Part model, mm, in its own coordinate system. Face numbers are marked on the shaded views. A direction names the side the tool comes from. Round coordinates to 2 decimals unless told otherwise and drop trailing zeros. Write each loop counter-clockwise with the first axis right and the second up, starting at its lowest first coordinate (ties: lowest second). Pieces come first, ordered by that corner, then holes. Notation, with made-up numbers: M -5.75,16 L 33.25,16 A30 ccw 33.25,38 Z; hole C 9.25,72.25 d7. An arc over 180 degrees is marked long. Use a Markdown table: item, result. Add a question column.
1) Slice it at D-D on y = 18. Write the cut outline in (x, z).
2) Drop flat-ended pins along their axis: P1, Ø1.5, axis at y = 25, z = 8, coming from the -X side; P2, Ø10, axis at y = -3.5, z = 8, coming from the +X side; P3, Ø12, axis at x = 19, y = 10, coming from the +Z side; P4, Ø1.5, axis at x = 31, z = 10.5, coming from the +Y side. Give the stop position or say it passes through.
3) Slice it at C-C on z = 26. Write the cut outline in (x, y), plus the area to 3 significant figures.
4) Two-plate mould, pull along Z, no slides. Class the marked faces 1, 2, 3 and 4: released by +Z, released by -Z, zero draft, split by the parting line, or undercut.
5) Slice it at A-A on z = 2.5. Write the cut outline in (x, y).
6) Slice it at B-B on y = 2. Write the cut outline in (x, z).
7) Which spindle directions (+Z, -Z, +X, -X, +Y, -Y) get a long thin tool onto all of the face, cutting with end or side? Do the marked faces 5, 6 and 7. Say none if no direction does.
8) Wall check: probe 1 along Z at (x, y) = (0, 0); probe 2 along Z at (x, y) = (0, 29.75); probe 3 along X at (y, z) = (-4.25, 8). Give the ranges that are in metal, low to high.
```python
from build123d import *

# Parameters (mm, degrees)
BOSS_EXTRUDE2_DEPTH       = 28
SKETCH5_R                 = 6
CUT_EXTRUDE1_DEPTH        = 24
CUT_EXTRUDE3_DEPTH        = 22
HOLE1_START               = 23.196151292
HOLE1_OUTLINE_R           = 3
HOLE1_DEPTH               = 12.803848708
HOLE1_START_2             = 32
HOLE1_2_OUTLINE_R         = 5
HOLE1_2_OUTLINE_R_2       = 3
HOLE1_2_DEPTH             = 4
F_6_0MM_DOWEL_HOLE2_D     = 6
F_6_0MM_DOWEL_HOLE2_DEPTH = 16
F_6_0MM_DOWEL_HOLE2_TIP   = 1.802581857
FILLET1_R                 = 3
SKETCH19_W                = 64
SKETCH19_H                = 4
BOSS_EXTRUDE3_DEPTH       = 2


# Read off the part's stored shape, not the designer's step: Hole1
with BuildPart() as part:
    # Sketch2 → Boss-Extrude2 (new body)
    with BuildSketch(Plane.XY):
        Polygon((0, -9), (-8, -9), (-8, 0), (-32, 0), (-32, 36), (32, 36), (32, 0), (8, 0), (8, -9), align=None)
    extrude(amount=BOSS_EXTRUDE2_DEPTH)

    # Sketch5 → Cut-Extrude1 (cut)
    with BuildSketch(Plane.XY):
        with Locations((0, 18)):
            Circle(SKETCH5_R)
    extrude(amount=CUT_EXTRUDE1_DEPTH, mode=Mode.SUBTRACT)

    # Sketch6 → Cut-Extrude3 (cut)
    with BuildSketch(Plane(origin=(0, 0, 0), x_dir=(-1, 0, 0), z_dir=(0, 0, -1))):
        with BuildLine():
            Line((-32, 36), (-32, 10))
            Line((-32, 10), (-27.5, 10))
            Line((-27.5, 10), (-14.77335007, 28.283390866))
            ThreePointArc((-14.77335007, 28.283390866), (-8.333635583, 33.954639387), (2.5e-08, 36))
            Line((2.5e-08, 36), (-32, 36))
        make_face()
        with BuildLine():
            Line((32, 36), (2.5e-08, 36))
            ThreePointArc((2.5e-08, 36), (8.333635604, 33.954639376), (14.77335007, 28.283390866))
            Line((14.77335007, 28.283390866), (27.5, 10))
            Line((27.5, 10), (32, 10))
            Line((32, 10), (32, 36))
        make_face()
    extrude(amount=-CUT_EXTRUDE3_DEPTH, mode=Mode.SUBTRACT)

    # Hole1 outline → Hole1 (cut)
    with BuildSketch(Plane(origin=(0, 0, 0), x_dir=(1, 0, 0), z_dir=(0, 1, 0)).offset(HOLE1_START)):
        with Locations((0, -11)):
            Circle(HOLE1_OUTLINE_R)
    extrude(amount=HOLE1_DEPTH, mode=Mode.SUBTRACT)

    # Hole1 2 outline → Hole1 2 (cut)
    with BuildSketch(Plane(origin=(0, 0, 0), x_dir=(1, 0, 0), z_dir=(0, 1, 0)).offset(HOLE1_START_2)):
        with Locations((0, -11)):
            Circle(HOLE1_2_OUTLINE_R)
        with Locations((0, -11)):
            Circle(HOLE1_2_OUTLINE_R_2, mode=Mode.SUBTRACT)
    extrude(amount=HOLE1_2_DEPTH, mode=Mode.SUBTRACT)

    # Ø6.0mm Dowel Hole2
    with Locations(Plane(origin=(0, -9, 0), x_dir=(-1, 0, 0), z_dir=(0, -1, 0))):
        with Locations((0, -20), (0, -8)):
            Hole(F_6_0MM_DOWEL_HOLE2_D / 2, depth=F_6_0MM_DOWEL_HOLE2_DEPTH)
            with Locations((0, 0, -(F_6_0MM_DOWEL_HOLE2_DEPTH + F_6_0MM_DOWEL_HOLE2_TIP / 2))):  # 118° drill point
                Cone(0, F_6_0MM_DOWEL_HOLE2_D / 2, F_6_0MM_DOWEL_HOLE2_TIP, mode=Mode.SUBTRACT)

    # Fillet1
    fillet1_edges = [part.edges().sort_by_distance(p)[0] for p in [
        (27.5, 10, 11),
        (-27.5, 10, 11),
    ]]
    fillet(fillet1_edges, radius=FILLET1_R)

    # Sketch19 → Boss-Extrude3 (add)
    with BuildSketch(Plane.XY.offset(28)):
        with Locations((0, 30)):
            Rectangle(SKETCH19_W, SKETCH19_H)
    extrude(amount=BOSS_EXTRUDE3_DEPTH)


solid = part.part
```
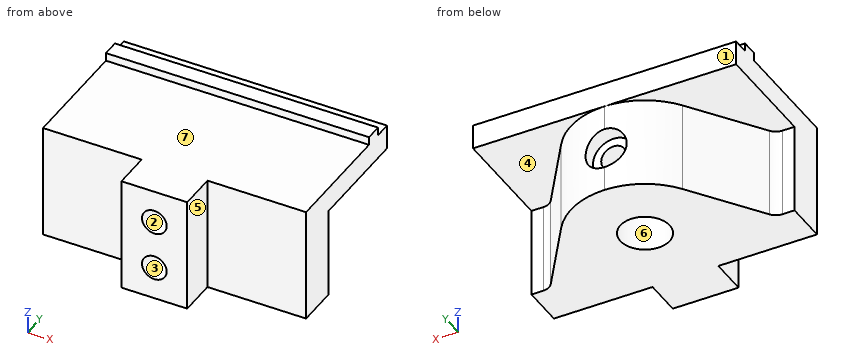
Entries:
| question | item | result |
|---|---|---|
| 1 | outline | M -32,22 L -21.93,22 L -21.93,0 L -6,0 L -6,24 L 6,24 L 6,0 L 21.93,0 L 21.93,22 L 32,22 L 32,28 L -32,28 Z |
| 2 | P1 | stops at x = -17.58 |
| 2 | P2 | stops at x = 32 |
| 2 | P3 | stops at z = 28 |
| 2 | P4 | stops at y = 10 |
| 3 | outline | M -32,0 L -8,0 L -8,-9 L 8,-9 L 8,0 L 32,0 L 32,36 L -32,36 Z |
| 3 | area | 2,450 mm^2 |
| 4 | face 1 | zero draft |
| 4 | face 2 | undercut |
| 4 | face 3 | undercut |
| 4 | face 4 | released by -Z |
| 5 | outline | M -32,0 L -8,0 L -8,-9 L 8,-9 L 8,0 L 32,0 L 32,10 L 29.07,10 A3 cw 26.6,11.29 L 14.77,28.28 A18 ccw -14.77,28.28 L -26.6,11.29 A3 cw -29.07,10 L -32,10 Z; hole C 0,18 d12 |
| 6 | outline | M -32,0 L 32,0 L 32,28 L -32,28 Z; hole C 0,8 d6; hole C 0,20 d6 |
| 7 | face 5 | +Z, -Z, +X, -Y |
| 7 | face 6 | -Z |
| 7 | face 7 | +Z, +X, -X, -Y |
| 8 | probe 1 | z = 0 to 5, 11 to 17, 23 to 28 |
| 8 | probe 2 | z = 0 to 8, 14 to 30 |
| 8 | probe 3 | x = -8 to -3, 3 to 8 |
